from build123d import *

# Parameters (mm, degrees)
F0_R     = 10.75
F0_R_2   = 10
F1_DEPTH = 2.5
F2_R     = 4.05
F3_DEPTH = 5.5
F4_SIZE  = 0.5
F5_R     = 4.55
F6_DEPTH = 2
F7_DEPTH = 0.5


# Not quite as in the source:
# - a feature names something its author has since deleted; it is built from what else it names


with BuildPart() as f1:
    # F0 (on Top) → F1 (new body)
    with BuildSketch(Plane.XY):
        Circle(F0_R)
        Circle(F0_R_2, mode=Mode.SUBTRACT)
        Circle(F0_R_2)
        Polygon((-0.8144098687, 5.5770273648), (3.432810713, 8.7260752933), (2.0940857055, 4.3571935282), (5.0940976108, -0.8390625077), (5.23705231, -2.0832140472), (5.8405975225, -7.3359389308), (2.7263974316, -3.992128183), (-3.2736025686, -3.992128183), (-4.4226424415, -3.4938133181), (-9.2734082358, -1.3901363628), (-4.8204831373, -0.3650653455), (-1.8204831373, 4.8310870772), align=None, mode=Mode.SUBTRACT)
        Polygon((2.0940857055, 4.3571935282), (3.432810713, 8.7260752933), (-0.8144098687, 5.5770273648), (-1.8204831373, 4.8310870772), (-4.8204831373, -0.3650653455), (-9.2734082358, -1.3901363628), (-4.4226424415, -3.4938133181), (-3.2736025686, -3.992128183), (2.7263974316, -3.992128183), (5.8405975225, -7.3359389308), (5.23705231, -2.0832140472), (5.0940976108, -0.8390625077), align=None)
    extrude(amount=F1_DEPTH)

    # F2 (on face) → F3 (join)
    with BuildSketch(Plane.XY.offset(2.5)):
        Circle(F2_R)
    extrude(amount=F3_DEPTH)

    # F4
    f4_edges = [f1.edges().sort_by_distance(p)[0] for p in [
        (-4.05, 0, 8),
    ]]
    chamfer(f4_edges, length=F4_SIZE)

    # F5 (on face) → F6 (join)
    with BuildSketch(Plane.XY.offset(2.5)):
        Circle(F5_R)
    extrude(amount=F6_DEPTH)

    # F0 (on Top) → F7 (cut)
    with BuildSketch(Plane.XY):
        Polygon((2.0940857055, 4.3571935282), (3.432810713, 8.7260752933), (-0.8144098687, 5.5770273648), (-1.8204831373, 4.8310870772), (-4.8204831373, -0.3650653455), (-9.2734082358, -1.3901363628), (-4.4226424415, -3.4938133181), (-3.2736025686, -3.992128183), (2.7263974316, -3.992128183), (5.8405975225, -7.3359389308), (5.23705231, -2.0832140472), (5.0940976108, -0.8390625077), align=None)
    extrude(amount=F7_DEPTH, mode=Mode.SUBTRACT)


solid = f1.part
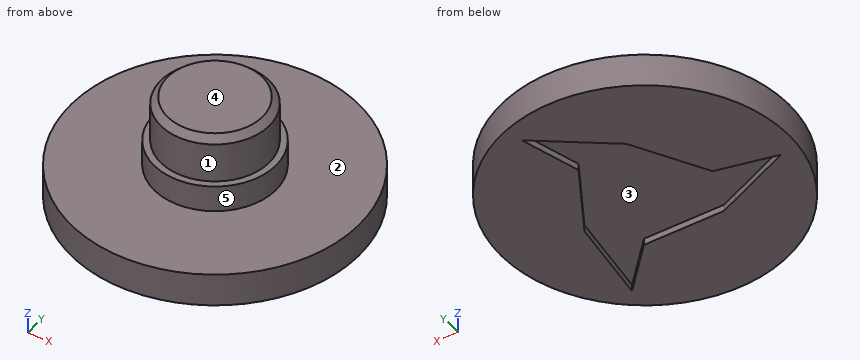
Input: part model. Units: mm. Frame: model coordinates. Face numbers are marked on the shaded views. A direction names the side the tool comes from. Coordinates: 2 decimals unless noted, no trailing zeros. Loops run counter-clockwise (first coordinate to the right, second up) from the corner with the lowest first, then second, coordinate; pieces in that order, holes last.
(1) Set-up query: the marked faces 4 and 5. Return all of +Z, -Z, +X, -X, +Y, -Y with unobstructed straight access to the full face (end or side cutting, diameter ignored); none if empty.
(2) Section D-D on x = 0. Return the cut outline in (y, z), then the cut area to 3 significant figures.
(3) Section A-A on x = -7.75. Return the cut outline in (y, z), then the cut area to 3 significant figures.
(4) Section B-B on y = 8. Return the cut outline in (x, z), then the cut area to 3 significant figures.
(5) Section C-C on z = 3. Return the cut outline in (x, y).
(6) First-contact query: pin 1 Ø11 at (x, y) = (-4.5, 3) entering from +Z; pin 2 Ø2 at (y, z) = (-1, 6) entering from +X; pin 3 Ø0.6 at (x, z) = (1, 0.5) entering from +Y; pin 4 Ø3 at (x, z) = (3.5, 1) entering from +Y. Flat tips, straight axial feed; report the tip coordinate or a pass-through.
(7) Pull-direction query (X, two-part tool) for the marked faces 1, 2 and 3; classes: released by +X, released by -X, zero draft, split by the parting line, or undercut.
(8) Material intervals for probe 1 along Z at (x, y) = (-0.25, 2.25); probe 2 along Z at (x, y) = (8.5, 4.5); probe 3 along X at (y, z) = (0.25, 4), sorted ascending.
Data:
1. face 4: +Z, +X, -X, +Y, -Y
1. face 5: +Z
2. outline: (-10.75, 0) - (-3.99, 0) - (-3.99, 0.5) - (6.18, 0.5) - (6.18, 0) - (10.75, 0) - (10.75, 2.5) - (4.55, 2.5) - (4.55, 4.5) - (4.05, 4.5) - (4.05, 7.5) - (3.55, 8) - (-3.55, 8) - (-4.05, 7.5) - (-4.05, 4.5) - (-4.55, 4.5) - (-4.55, 2.5) - (-10.75, 2.5) - close
2. area: 95.0 mm2
3. outline: (-7.45, 0) - (-2.05, 0) - (-2.05, 0.5) - (-1.04, 0.5) - (-1.04, 0) - (7.45, 0) - (7.45, 2.5) - (-7.45, 2.5) - close
3. area: 36.7 mm2
4. outline: (-7.18, 0) - (2.45, 0) - (2.45, 0.5) - (3.21, 0.5) - (3.21, 0) - (7.18, 0) - (7.18, 2.5) - (-7.18, 2.5) - close
4. area: 35.5 mm2
5. outline: circle Ø9.1 at (0, 0)
6. pin 1: stops at z = 8
6. pin 2: stops at x = 4.05
6. pin 3: stops at y = 10.73
6. pin 4: stops at y = 10.56
7. face 1: split by the parting line
7. face 2: zero draft
7. face 3: undercut
8. probe 1: z = 0.5 to 8
8. probe 2: z = 0 to 2.5
8. probe 3: x = -4.54 to 4.54
